Design review of the part built by this model. Coordinates are the model's own, in mm. A direction names the side the tool comes from. Round coordinates to 2 decimals unless told otherwise and drop trailing zeros. Loops run counter-clockwise (first coordinate to the right, second up) from the corner with the lowest first, then second, coordinate; pieces in that order, holes last. Notation, with made-up numbers: (23, 83) - (82, 83) arc R28 ccw to (82, 112) - close; hole circle Ø6 at (66.5, -4). An arc over 180 degrees is marked (long way). Return JSON: item names as keys, results as strings. Group by question number.
(1) The part is to be moulded in two halves that separate along Y. For faces 1 (the cylindrical face through (6, 46, 8)), 2 (the flat face through (5, 24, 10)), 3 (the cylindrical face through (4.675, 35.536, 5.07)), say which applies: pulls with the +Y half, pulls with the -Y half, needs draft (parallel to the pull), parting line crosses it, or undercut.
(2) For faces 4 (the flat face through (5, 47, 2)), 5 (the flat face through (6, 13, 6)), list the 3-axis set-ups (+Z, -Z, +X, -X, +Y, -Y) from which the entire face can be reached by the end or side of a thin tool; tool diameter is ignored.
(3) We need section D-D, the plane y = 11.5. Write out the cut boundary in (x, z).
(4) We need section C-C, the plane z = 1.5. Write out the cut boundary in (x, y).
(5) We need section A-A, the plane y = 37. Write out the cut boundary in (x, z).
(6) Wall thickness on L1, parallel to Y at x = 5, z = 1.25; L2, parallel to Y at x = 5.5, z = 9; L3, parallel to X at y = 13, z = 8: over which ranges is each line inside the solid? List them lowest first. Write a range as [from, to].
(7) We need section B-B, the plane x = 5. Write out the cut boundary in (y, z), and give its area (3 significant figures).
from build123d import *

# Parameters (mm, degrees)
SKETCH1_W           = 10
SKETCH1_H           = 47
BOSS_EXTRUDE1_DEPTH = 10
SKETCH2_R           = 1.5
CUT_EXTRUDE1_DEPTH  = 10
FILLET1_R           = 5
SKETCH3_W           = 10
SKETCH3_H           = 47
CUT_EXTRUDE2_DEPTH  = 1
SKETCH4_R           = 6.5
CUT_EXTRUDE3_DEPTH  = 22
SKETCH5_R           = 3
CUT_EXTRUDE4_DEPTH  = 4


with BuildPart() as part:
    # Sketch1 → Boss-Extrude1 (new body)
    with BuildSketch(Plane.XY):
        with Locations((5, 23.5)):
            Rectangle(SKETCH1_W, SKETCH1_H)
    extrude(amount=BOSS_EXTRUDE1_DEPTH)

    # Sketch2 → Cut-Extrude1 (cut)
    with BuildSketch(Plane.XY.offset(10)):
        with Locations((5, 37)):
            Circle(SKETCH2_R)
        with Locations((5, 11.5)):
            Circle(SKETCH2_R)
    extrude(amount=-CUT_EXTRUDE1_DEPTH, mode=Mode.SUBTRACT)

    # Fillet1
    fillet1_edges = [part.edges().sort_by_distance(p)[0] for p in [
        (5, 47, 10),
    ]]
    fillet(fillet1_edges, radius=FILLET1_R)

    # Sketch3 → Cut-Extrude2 (cut)
    with BuildSketch(Plane.ZY):
        with Locations((5, 23.5)):
            Rectangle(SKETCH3_W, SKETCH3_H)
    extrude(amount=-CUT_EXTRUDE2_DEPTH, mode=Mode.SUBTRACT)

    # Sketch4 → Cut-Extrude3 (cut)
    with BuildSketch(Plane.ZY.offset(-1)):
        with Locations((10, 0)):
            Circle(SKETCH4_R)
    extrude(amount=-CUT_EXTRUDE3_DEPTH, mode=Mode.SUBTRACT)

    # Sketch5 → Cut-Extrude4 (cut)
    with BuildSketch(Plane.XY.offset(10)):
        with Locations((5, 11.5)):
            Circle(SKETCH5_R)
    extrude(amount=-CUT_EXTRUDE4_DEPTH, mode=Mode.SUBTRACT)


solid = part.part
Solutions:
{
 "1": {"face 1": "pulls with the +Y half", "face 2": "needs draft", "face 3": "undercut"},
 "2": {"face 4": "+Z, -Z, +X, -X, +Y", "face 5": "+Z"},
 "3": {"outline": "(1, 0) - (3.5, 0) - (3.5, 6) - (2, 6) - (2, 10) - (1, 10) - close; (6.5, 0) - (10, 0) - (10, 10) - (8, 10) - (8, 6) - (6.5, 6) - close"},
 "4": {"outline": "(1, 0) - (10, 0) - (10, 47) - (1, 47) - close; hole circle Ø3 at (5, 11.5); hole circle Ø3 at (5, 37)"},
 "5": {"outline": "(1, 0) - (3.5, 0) - (3.5, 10) - (1, 10) - close; (6.5, 0) - (10, 0) - (10, 10) - (6.5, 10) - close"},
 "6": {"L1": "[0, 10], [13, 35.5], [38.5, 47]", "L2": "[6.42, 8.54], [14.46, 35.59], [38.41, 45]", "L3": "[1, 2.4], [7.6, 10]"},
 "7": {"outline": "(0, 0) - (10, 0) - (10, 6) - (8.5, 6) - (8.5, 10) - (6.5, 10) arc R6.5 cw to (0, 3.5) - close; (13, 0) - (35.5, 0) - (35.5, 10) - (14.5, 10) - (14.5, 6) - (13, 6) - close; (38.5, 0) - (47, 0) - (47, 5) arc R5 ccw to (42, 10) - (38.5, 10) - close", "area": "359 mm^2"}
}
